Model file for the job. Use its own axes, mm. Face numbers are marked on the shaded views. A direction names the side the tool comes from. Round coordinates to 2 decimals unless told otherwise and drop trailing zeros. Order: outer loops, then holes, each group sorted by start corner. A loop starts at its lowest first (then second) coordinate and runs counter-clockwise, first axis right, second up. Notation, with made-up numbers: (34.5, 80.25) -> (63.5, 80.25) arc R16 ccw to (63.5, 87.25) -> close; hole circle Ø3 at (16.5, 46). An arc over 180 degrees is marked (long way). Put each result on its own line as item: value. Start each with the question number.
Q1. 3-axis set-ups, long thin cutter, end or side, ignore diameter. For the marked faces 4, 5 and 6: which of +Z, -Z, +X, -X, +Y, -Y reach the whole face in a straight line?
Q2. Cut at B-B, the plane z = 18.5. List the corners of the cut face in (x, y), and give its area (3 significant figures).
Q3. Pull direction Y, two halves, no side cores. Call the marked faces 1, 2 and 3: released by +Y, released by -Y, zero draft, split by the parting line, or undercut.
Q4. Probe L1, parallel to Y at x = 0, z = 6.25; L2, parallel to X at y = 8, z = 46.5; L3, parallel to Y at x = -3.5, z = 10. List the from-to ranges inside material, lowest first.
Q5. Flat gauge pins, fed straight in: P1, Ø2, axis at x = 12, y = 1, coming from the +Z side; P2, Ø1, axis at x = -5, z = 42.5, coming from the +Y side; P3, Ø12, axis at x = -9.5, z = 25, coming from the -Y side. Where does each tip first touch, or does it go through?
Q6. Cut at A-A, the plane z = 63. List the corners of the cut face in (x, y), and give its area (3 significant figures).
from build123d import *

# Parameters (mm, degrees)
F0_R         = 13.97
F1_DEPTH     = 38.1
F2_R         = 15.24
F3_DEPTH     = 12.7
F4_R         = 8.89
F5_DEPTH     = 7.62
F6_R         = 6.35
F7_DEPTH     = 10.16
F8_R         = 4.826
F9_DEPTH     = 25.4
F10_S5_R     = 8.89
F10_T6_DEPTH = 23
F12_D        = 20.32
F12_DEPTH    = 7.62
F12_TIP      = 6.1047438893


# Not quite as in the source:
# - a fillet or chamfer that OpenCascade refuses, or shapes differently, is made with other operations: its cross-section is extruded or revolved along the edge and cut away or added


with BuildPart() as f1:
    # F0 (on Top) → F1 (new body)
    with BuildSketch(Plane.XY):
        Circle(F0_R)
    extrude(amount=F1_DEPTH)

    # F2 (on face) → F3 (join)
    with BuildSketch(Plane.XY.offset(38.1)):
        Circle(F2_R)
    extrude(amount=F3_DEPTH)

    # F4 (on face) → F5 (join)
    with BuildSketch(Plane.XY.offset(50.8)):
        Circle(F4_R)
    extrude(amount=F5_DEPTH)

    # F6 (on face) → F7 (join)
    with BuildSketch(Plane.XY.offset(58.42)):
        Circle(F6_R)
    extrude(amount=F7_DEPTH)

    # F8 (on face) → F9 (join)
    with BuildSketch(Plane.XY.offset(68.58)):
        Circle(F8_R)
    extrude(amount=F9_DEPTH)

    # F10: chamfer of 6.604 on 1 edges, made by hand


with BuildPart() as f10_tool2:
    # F10_s3 → F10_t4 (revolve)
    with BuildSketch(Plane.XZ):
        Polygon((15.24, 44.196), (8.636, 50.8), (15.24, 50.8), align=None)
    revolve(axis=Axis((0, 0, 50.8), (0, 0, 1)))

    # F10_s5 → F10_t6 (cut, symmetric)
    with BuildSketch(Plane.XY.offset(47.5)):
        Circle(F10_S5_R)
    extrude(amount=F10_T6_DEPTH, both=True, mode=Mode.SUBTRACT)


with BuildPart() as f1_1:
    add(f1.part)

    # F10_t1: cut F10_tool2
    add(f10_tool2.part, mode=Mode.SUBTRACT)

    # F12
    with Locations(Plane(origin=(0, 0, 0), x_dir=(1, 0, 0), z_dir=(0, 0, -1))):
        with Locations((0, 0)):
            Hole(F12_D / 2, depth=F12_DEPTH)
            with Locations((0, 0, -(F12_DEPTH + F12_TIP / 2))):  # 118° drill point
                Cone(0, F12_D / 2, F12_TIP, mode=Mode.SUBTRACT)


solid = f1_1.part
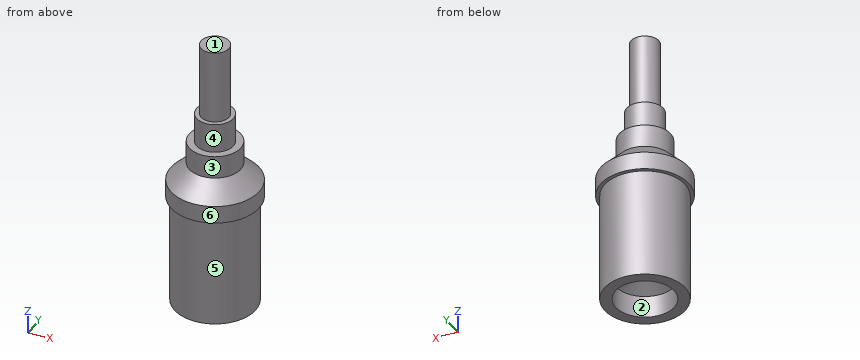
Ans:
1. face 4: +Z
1. face 5: -Z
1. face 6: +Z, -Z
2. outline: circle Ø27.94 at (0, 0)
2. area: 613 mm^2
3. face 1: zero draft
3. face 2: undercut
3. face 3: split by the parting line
4. L1: y = -13.97 to -10.16, 10.16 to 13.97
4. L2: x = -10.17 to 10.17
4. L3: y = -13.52 to -5.12, 5.12 to 13.52
5. P1: stops at z = 48.39
5. P2: stops at y = 14.56
5. P3: stops at y = -13.52
6. outline: circle Ø12.7 at (0, 0)
6. area: 127 mm^2
